Input: part model. Units: mm. Frame: model coordinates. A direction names the side the tool comes from. Coordinates: 2 decimals unless noted, no trailing zeros. Loops run counter-clockwise (first coordinate to the right, second up) from the corner with the lowest first, then second, coordinate; pieces in that order, holes last. Notation, with made-up numbers: (40, 46) - (87, 46) arc R28 cw to (87, 74) - close; hole circle Ø7 at (65, 19.5). An arc over 180 degrees is marked (long way). Use one line per item in the form item = value.
Autodesk Fusion 360 part; units mm, degrees
sketch "Skizze1" plane through (0, 0, 0) normal (0, 1, 0) x (1, 0, 0)
  line L0 (10, 0) -> (136, 0)
  line L1 (146, -10) -> (146, -173)
  line L2 (136, -183) -> (10, -183)
  line L3 (0, -173) -> (0, -10)
  line L4 (20, -20) -> (126, -20)
  line L5 (126, -20) -> (126, -163)
  line L6 (126, -163) -> (20, -163)
  line L7 (20, -163) -> (20, -20)
  circle A0 centre (10, -30) radius 3
  circle A1 centre (10, -153) radius 3
  circle A2 centre (136, -30) radius 3
  circle A3 centre (136, -153) radius 3
  circle A4 centre (28.55, -80) radius 2.25
  line L8 (120.45, -77.5) -> (114.45, -77.5)
  arc A5 (114.45, -77.5) -> (114.45, -82.5) centre (114.45, -80) ccw
  line L9 (114.45, -82.5) -> (120.45, -82.5)
  arc A6 (120.45, -82.5) -> (120.45, -77.5) centre (120.45, -80) ccw
  line L10 (120.45, -80) -> (114.45, -80) construction
  circle A7 centre (73, -80) radius 4
  arc A8 (10, 0) -> (0, -10) centre (10, -10) ccw
  arc A9 (146, -10) -> (136, 0) centre (136, -10) ccw
  arc A10 (0, -173) -> (10, -183) centre (10, -173) ccw
  arc A11 (136, -183) -> (146, -173) centre (136, -173) ccw
  point P0 (146, 0)
  point P1 (0, -183)
  point P2 (117.45, -80)
  dimension "d1" = 183
  dimension "d2" = 146
  dimension "d3" = 20
  dimension "d4" = 20
  dimension "d5" = 20
  dimension "d6" = 20
  dimension "d7" = 6
  dimension "d8" = 6
  dimension "d9" = 6
  dimension "d10" = 6
  dimension "d11" = 10
  dimension "d12" = 10
  dimension "d13" = 30
  dimension "d14" = 30
  dimension "d15" = 30
  dimension "d16" = 10
  dimension "d17" = 10
  dimension "d18" = 30
  dimension "d19" = 4.5
  dimension "d22" = 8.55
  dimension "d24" = 6
  dimension "d25" = 5
  dimension "d26" = 88.9
  dimension "d27" = 60
  dimension "d28" = 60
  dimension "d30" = 8
  dimension "d31" = 44.45
  dimension "d32" = 60
  dimension "d35" = 10
extrude "Extrusion1" add sketch "Skizze1" along normal blind 5 contours L0 L1 L2 L3 A8 A9 A10 A11 | L4 L5 L6 L7
Q1. Pull-direction query (X, two-part tool) for faces 1 (the flat face through (0, 2, 93)), 2 (the cylindrical face through (142.99, 2.46, 2.85)), 3 (the cylindrical face through (12.77, 2.46, 28.85)); classes: pulls with the +X half, pulls with the -X half, needs draft (parallel to the pull), parting line crosses it, or undercut.
Check values:
face_1 = pulls with the -X half
face_2 = pulls with the +X half
face_3 = undercut
Q2. Ray query, line 1 along X through (y, z) = (2, 153); line 2 along Z through (x, y) = (136, 2.25); line 3 along X through (y, z) = (3.7, 80). Return the intervals inside material, ascending. Write a range as [from, to].
Check values:
line_1 = [0, 7], [13, 133], [139, 146]
line_2 = [0, 27], [33, 150], [156, 183]
line_3 = [0, 26.3], [30.8, 69], [77, 111.95], [122.95, 146]
Q3. Cut plane B-B, the plane x = 73. Return loops of the section in (y, z), then the cut area to 3 significant figures.
Check values:
outline = (0, 0) - (5, 0) - (5, 76) - (0, 76) - close; (0, 84) - (5, 84) - (5, 183) - (0, 183) - close
area = 875 mm²
Q4. Cut plane A-A, the plane z = 80. Return loops of the section in (x, y).
Check values:
outline = (0, 0) - (26.3, 0) - (26.3, 5) - (0, 5) - close; (30.8, 0) - (69, 0) - (69, 5) - (30.8, 5) - close; (77, 0) - (111.95, 0) - (111.95, 5) - (77, 5) - close; (122.95, 0) - (146, 0) - (146, 5) - (122.95, 5) - close
Q5. Set-up query: faces 4 (the cylindrical face through (122.95, 2.46, 79.95)), 5 (the flat face through (72, 2, 0)). Return all of +Z, -Z, +X, -X, +Y, -Y with unobstructed straight access to the full face (end or side cutting, diameter ignored); none if empty.
Check values:
face_4 = +Y, -Y
face_5 = -Z, +X, -X, +Y, -Y
